Source: CAD feature listing. Evaluate the final solid. Frame: model axes, mm. Round coordinates to 2 decimals unless told otherwise and drop trailing zeros. Order: outer loops, then holes, each group sorted by start corner. A loop starts at its lowest first (then second) coordinate and runs counter-clockwise, first axis right, second up.
Autodesk Inventor part; units mm, degrees
ref_plane "YZ Plane" through (0, 0, 0) normal (1, 0, 0) x (0, 1, 0)
ref_plane "XZ Plane" through (0, 0, 0) normal (0, 1, 0) x (-1, 0, 0)
ref_plane "XY Plane" through (0, 0, 0) normal (0, 0, 1) x (1, 0, 0)
sketch "Sketch1" plane through (0, 0, 0) normal (0, 0, 1) x (1, 0, 0)
  line L0 (0, 0) -> (0, 3) construction
  line L1 (0, 3) -> (50, 3)
  line L2 (50, 3) -> (50, 0)
  line L3 (50, 0) -> (100, 0)
  line L4 (100, 0) -> (100, 3)
  line L5 (100, 3) -> (160, 3)
  line L6 (160, 3) -> (160, 0)
  line L7 (160, 0) -> (210, 0)
  line L8 (210, 0) -> (210, 3)
  line L9 (210, 3) -> (260, 3)
  line L10 (260, 3) -> (260, 33)
  line L11 (260, 33) -> (257, 33)
  line L12 (257, 33) -> (257, 53)
  line L13 (257, 53) -> (260, 53)
  line L14 (260, 53) -> (260, 86)
  line L15 (0, 86) -> (0, 53)
  line L16 (0, 53) -> (3, 53)
  line L17 (3, 53) -> (3, 33)
  line L18 (3, 33) -> (0, 33)
  line L19 (0, 33) -> (0, 3)
  line L20 (260, 0) -> (260, 25) construction
  line L21 (260, 25) -> (260, 28) construction
  line L22 (135, 28) -> (135, 0) construction
  line L23 (135, 0) -> (135, 20) construction
  line L24 (130, 28) -> (130, 0) construction
  line L25 (130, 0) -> (130, 25) construction
  line L26 (260, 0) -> (260, 22) construction
  line L27 (260, 22) -> (260, 32) construction
  line L28 (260, 32) -> (145, 32) construction
  line L29 (145, 32) -> (130, 32) construction
  line L30 (130, 32) -> (130, 22)
  line L31 (145, 22) -> (145, 32)
  line L32 (130, 32) -> (145, 32)
  line L33 (130, 22) -> (145, 22)
  line L34 (260, 86) -> (210, 86)
  line L35 (210, 86) -> (210, 83)
  line L36 (100, 86) -> (100, 83)
  line L37 (100, 83) -> (50, 83)
  line L38 (50, 83) -> (50, 86)
  line L39 (50, 86) -> (0, 86)
  line L40 (260, 83) -> (193, 83) construction
  line L41 (193, 83) -> (193, 77)
  line L42 (193, 77) -> (133, 77)
  line L43 (133, 77) -> (133, 86)
  line L44 (210, 83) -> (193, 83)
  line L45 (133, 86) -> (100, 86)
  line L46 (145, 32) -> (170, 32) construction
  line L47 (170, 32) -> (170, 0) construction
  line L48 (170, 0) -> (170, 40) construction
  line L49 (170, 40) -> (170, 50)
  line L50 (170, 50) -> (185, 50)
  line L51 (185, 50) -> (185, 40)
  line L52 (185, 40) -> (170, 40)
  point P0 (0, 18)
  dimension "d0" = 3
  dimension "d2" = 50
  dimension "d3" = 60
  dimension "d4" = 50
  dimension "d5" = 50
  dimension "d6" = 30
  dimension "d7" = 3
  dimension "d8" = 20
  dimension "d9" = 33
  dimension "d10" = 33
  dimension "d11" = 3
  dimension "d12" = 20
  dimension "d24" = 20
  dimension "d29" = 25
  dimension "d32" = 22
  dimension "d33" = 10
  dimension "d34" = 115
  dimension "d35" = 15
  dimension "d37" = 3
  dimension "d40" = 50
  dimension "d41" = 50
  dimension "d42" = 67
  dimension "d43" = 6
  dimension "d44" = 60
  dimension "d45" = 25
  dimension "d46" = 40
  dimension "d47" = 10
  dimension "d48" = 15
extrude "Extrusion1" add sketch "Sketch1" along normal blind 3
properties part number "Belakang"
1. Section B-B on y = 79.5. Return loops of the section in (x, z).
2. Section C-C on z = 0.95. State how many separate pieces and enclosed holes the cut face has, plus the area to 3 significant figures.
3. First-contact query: pin 1 (1.5 mm diameter, centred on x = 1, z = 1, fed in from -Y); pin 2 (1.5 mm diameter, centred on x = 198.5, z = 2, fed in from +Y). Flat tips, straight axial feed; report the tip coordinate or a pass-through.
4. Line query: line 1 along Y through (x, z) = (139, 1.55); line 2 along Y through (x, z) = (194, 1.45); line 3 along Y through (x, z) = (150.5, 2.45). Output: solid intervals per line, ascending.
5. Section D-D on x = 219. Return loops of the section in (y, z), plus the area to 3 significant figures.
6. Section A-A on x = 142. Return loops of the section in (y, z).
Result:
1. outline: (0, 0) - (133, 0) - (133, 3) - (0, 3) - close; (193, 0) - (260, 0) - (260, 3) - (193, 3) - close
2. separate pieces: 1
2. enclosed holes: 2
2. area: 20,700 mm2
3. pin 1: stops at y = 3
3. pin 2: stops at y = 83
4. line 1: y = 3 to 22, 32 to 77
4. line 2: y = 0 to 83
4. line 3: y = 3 to 77
5. outline: (3, 0) - (86, 0) - (86, 3) - (3, 3) - close
5. area: 249 mm2
6. outline: (3, 0) - (22, 0) - (22, 3) - (3, 3) - close; (32, 0) - (77, 0) - (77, 3) - (32, 3) - close
